For this review, take the finished solid that the model builds, in its own axes (mm). Face numbers are marked on the shaded views. A direction names the side the tool comes from. Coordinates: 2 decimals unless noted, no trailing zeros. Loops run counter-clockwise (first coordinate to the right, second up) from the corner with the lowest first, then second, coordinate; pieces in that order, holes last. Notation, with made-up numbers: M 15.25,-21.75 L 42.25,-21.75 A24 cw 42.25,10.25 Z; hole C 48.5,63 d9. An arc over 180 degrees is marked long. Write item = value, one per line.
from build123d import *

# Parameters (mm, degrees)
ESQUISSE1_W                       = 5.5
ESQUISSE1_H                       = 36
BOSS_EXTRU_1_DEPTH                = 10
ESQUISSE2_R                       = 1.7
ENL_V_MAT_EXTRU_1_DEPTH           = 4
ENL_V_MAT_EXTRU_2_DEPTH           = 3.5
ENL_V_MAT_EXTRU_2_DRAFT           = 5
ENL_V_MAT_EXTRU_2_PROFILE_2_DEPTH = 3.5
ENL_V_MAT_EXTRU_2_PROFILE_2_DRAFT = 5
ENL_V_MAT_EXTRU_2_PROFILE_3_DEPTH = 3.5
ENL_V_MAT_EXTRU_2_PROFILE_3_DRAFT = 5
ENL_V_MAT_EXTRU_2_PROFILE_4_DEPTH = 3.5
ENL_V_MAT_EXTRU_2_PROFILE_4_DRAFT = 5
ESQUISSE4_W                       = 9.5
ESQUISSE4_H                       = 5
BOSS_EXTRU_2_DEPTH                = 50
ESQUISSE5_W                       = 9.5
ESQUISSE5_H                       = 9.5
BOSS_EXTRU_3_DEPTH                = 32
CONG_1_R                          = 4.75


with BuildPart() as part:
    # Esquisse1 → Boss.-Extru.1 (new body)
    with BuildSketch(Plane.XY):
        Rectangle(ESQUISSE1_W, ESQUISSE1_H)
    extrude(amount=BOSS_EXTRU_1_DEPTH)

    # Esquisse2 → Enlèv. mat.-Extru.1 (cut)
    with BuildSketch(Plane(origin=(2.75, 0, 0), x_dir=(0, 0, -1), z_dir=(1, 0, 0))):
        with Locations((-4, 10)):
            Circle(ESQUISSE2_R)
        with Locations((-4, 2)):
            Circle(ESQUISSE2_R)
        with Locations((-4, -6)):
            Circle(ESQUISSE2_R)
        with Locations((-4, -14)):
            Circle(ESQUISSE2_R)
    extrude(amount=-ENL_V_MAT_EXTRU_1_DEPTH, mode=Mode.SUBTRACT)


with BuildPart() as enl_v_mat_extru_2_tool:
    # Esquisse3 → Enlèv. mat.-Extru.2 (with draft: the straight prism first)
    with BuildSketch(Plane(origin=(-2.75, 0, 0), x_dir=(0, 0, -1), z_dir=(1, 0, 0))):
        Polygon((-2.574135551, 4.901765653), (-5.800070547, 4.685717662), (-7.225934996, 1.783952009), (-5.425864449, -0.901765653), (-2.199929453, -0.685717662), (-0.774065004, 2.216047991), align=None)
    extrude(amount=ENL_V_MAT_EXTRU_2_DEPTH)
    # Enlèv. mat.-Extru.2: the draft: its side faces are tilted about the plane it starts from
    enl_v_mat_extru_2_sides = [enl_v_mat_extru_2_tool.faces().sort_by_distance(p)[0] for p in [
        (-1, 4.793741658, 4.187103049),
        (-1, 3.234834835, 6.513002771),
        (-1, 0.441093178, 6.325899723),
        (-1, -0.793741658, 3.812896951),
        (-1, 0.765165165, 1.486997229),
        (-1, 3.558906822, 1.674100277),
    ]]
    draft(enl_v_mat_extru_2_sides, Plane(origin=(-2.75, 0, 0), x_dir=(0, 0, -1), z_dir=(1, 0, 0)), ENL_V_MAT_EXTRU_2_DRAFT)


with BuildPart() as part_1:
    add(part.part)

    # Enlèv. mat.-Extru.2: cut by enl_v_mat_extru_2_tool
    add(enl_v_mat_extru_2_tool.part, mode=Mode.SUBTRACT)


with BuildPart() as enl_v_mat_extru_2_profile_2_tool:
    # Esquisse3 → Enlèv. mat.-Extru.2 profile 2 (with draft: the straight prism first)
    with BuildSketch(Plane(origin=(-2.75, 0, 0), x_dir=(0, 0, -1), z_dir=(1, 0, 0))):
        Polygon((-2.574135551, 12.901765653), (-5.800070547, 12.685717662), (-7.225934996, 9.783952009), (-5.425864449, 7.098234347), (-2.199929453, 7.314282338), (-0.774065004, 10.216047991), align=None)
    extrude(amount=ENL_V_MAT_EXTRU_2_PROFILE_2_DEPTH)
    # Enlèv. mat.-Extru.2 profile 2: the draft: its side faces are tilted about the plane it starts from
    enl_v_mat_extru_2_profile_2_sides = [enl_v_mat_extru_2_profile_2_tool.faces().sort_by_distance(p)[0] for p in [
        (-1, 12.793741658, 4.187103049),
        (-1, 11.234834835, 6.513002771),
        (-1, 8.441093178, 6.325899723),
        (-1, 7.206258342, 3.812896951),
        (-1, 8.765165165, 1.486997229),
        (-1, 11.558906822, 1.674100277),
    ]]
    draft(enl_v_mat_extru_2_profile_2_sides, Plane(origin=(-2.75, 0, 0), x_dir=(0, 0, -1), z_dir=(1, 0, 0)), ENL_V_MAT_EXTRU_2_PROFILE_2_DRAFT)


with BuildPart() as part_2:
    add(part_1.part)

    # Enlèv. mat.-Extru.2 profile 2: cut by enl_v_mat_extru_2_profile_2_tool
    add(enl_v_mat_extru_2_profile_2_tool.part, mode=Mode.SUBTRACT)


with BuildPart() as enl_v_mat_extru_2_profile_3_tool:
    # Esquisse3 → Enlèv. mat.-Extru.2 profile 3 (with draft: the straight prism first)
    with BuildSketch(Plane(origin=(-2.75, 0, 0), x_dir=(0, 0, -1), z_dir=(1, 0, 0))):
        Polygon((-2.574135551, -3.098234347), (-5.800070547, -3.314282338), (-7.225934996, -6.216047991), (-5.425864449, -8.901765653), (-2.199929453, -8.685717662), (-0.774065004, -5.783952009), align=None)
    extrude(amount=ENL_V_MAT_EXTRU_2_PROFILE_3_DEPTH)
    # Enlèv. mat.-Extru.2 profile 3: the draft: its side faces are tilted about the plane it starts from
    enl_v_mat_extru_2_profile_3_sides = [enl_v_mat_extru_2_profile_3_tool.faces().sort_by_distance(p)[0] for p in [
        (-1, -3.206258342, 4.187103049),
        (-1, -4.765165165, 6.513002771),
        (-1, -7.558906822, 6.325899723),
        (-1, -8.793741658, 3.812896951),
        (-1, -7.234834835, 1.486997229),
        (-1, -4.441093178, 1.674100277),
    ]]
    draft(enl_v_mat_extru_2_profile_3_sides, Plane(origin=(-2.75, 0, 0), x_dir=(0, 0, -1), z_dir=(1, 0, 0)), ENL_V_MAT_EXTRU_2_PROFILE_3_DRAFT)


with BuildPart() as part_3:
    add(part_2.part)

    # Enlèv. mat.-Extru.2 profile 3: cut by enl_v_mat_extru_2_profile_3_tool
    add(enl_v_mat_extru_2_profile_3_tool.part, mode=Mode.SUBTRACT)


with BuildPart() as enl_v_mat_extru_2_profile_4_tool:
    # Esquisse3 → Enlèv. mat.-Extru.2 profile 4 (with draft: the straight prism first)
    with BuildSketch(Plane(origin=(-2.75, 0, 0), x_dir=(0, 0, -1), z_dir=(1, 0, 0))):
        Polygon((-2.574135551, -11.098234347), (-5.800070547, -11.314282338), (-7.225934996, -14.216047991), (-5.425864449, -16.901765653), (-2.199929453, -16.685717662), (-0.774065004, -13.783952009), align=None)
    extrude(amount=ENL_V_MAT_EXTRU_2_PROFILE_4_DEPTH)
    # Enlèv. mat.-Extru.2 profile 4: the draft: its side faces are tilted about the plane it starts from
    enl_v_mat_extru_2_profile_4_sides = [enl_v_mat_extru_2_profile_4_tool.faces().sort_by_distance(p)[0] for p in [
        (-1, -11.206258342, 4.187103049),
        (-1, -12.765165165, 6.513002771),
        (-1, -15.558906822, 6.325899723),
        (-1, -16.793741658, 3.812896951),
        (-1, -15.234834835, 1.486997229),
        (-1, -12.441093178, 1.674100277),
    ]]
    draft(enl_v_mat_extru_2_profile_4_sides, Plane(origin=(-2.75, 0, 0), x_dir=(0, 0, -1), z_dir=(1, 0, 0)), ENL_V_MAT_EXTRU_2_PROFILE_4_DRAFT)


with BuildPart() as part_4:
    add(part_3.part)

    # Enlèv. mat.-Extru.2 profile 4: cut by enl_v_mat_extru_2_profile_4_tool
    add(enl_v_mat_extru_2_profile_4_tool.part, mode=Mode.SUBTRACT)

    # Esquisse4 → Boss.-Extru.2 (add)
    with BuildSketch(Plane.XY.offset(10)):
        with Locations((2, 2.5)):
            Rectangle(ESQUISSE4_W, ESQUISSE4_H)
    extrude(amount=BOSS_EXTRU_2_DEPTH)

    # Esquisse5 → Boss.-Extru.3 (add)
    with BuildSketch(Plane.XZ):
        with Locations((2, 55.25)):
            Rectangle(ESQUISSE5_W, ESQUISSE5_H)
    extrude(amount=BOSS_EXTRU_3_DEPTH)

    # Congé1
    cong_1_edges = [part_4.edges().sort_by_distance(p)[0] for p in [
        (-2.75, -32, 55.25),
        (2, -32, 50.5),
        (6.75, -32, 55.25),
        (2, -32, 60),
    ]]
    fillet(cong_1_edges, radius=CONG_1_R - 0.0001)  # a hair under: the kernel refuses the full size


solid = part_4.part
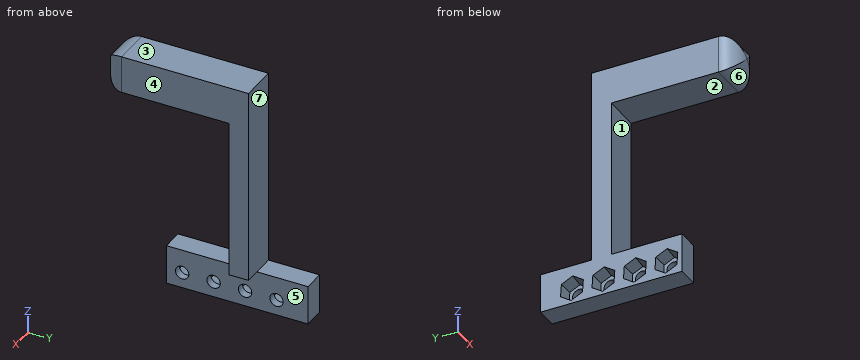
Q1. Draft analysis for pull direction Z (two halves, no side actions). For the marked faces 1, 2, 3 and 4, state which applies: +Z half, -Z half, draft (parallel to the pull), parting line (faces both ways), or undercut.
Solved:
face_1 = undercut
face_2 = undercut
face_3 = +Z half
face_4 = draft
Q2. Add section C-C (z = 52.5). Write out the cut boundary in (x, y), and give its area (3 significant figures).
Solved:
outline = M -2.75,-27.25 A4.75 ccw -0.75,-31.12 L 4.75,-31.12 A4.75 ccw 6.75,-27.25 L 6.75,5 L -2.75,5 Z
area = 339 mm²
Q3. For line 1 along Y through (x, z) = (1.5, 4); line 2 along Y through (x, z) = (1.5, 3); line 3 along Z through (x, y) = (-2, -10.5), list the stretches that pass through material, from the lowest coordinate up.
Solved:
line_1 = -18 to -15.7, -12.3 to -7.7, -4.3 to 0.3, 3.7 to 8.3, 11.7 to 18
line_2 = -18 to -15.37, -12.63 to -7.37, -4.63 to 0.63, 3.37 to 8.63, 11.37 to 18
line_3 = 0 to 10, 50.5 to 60
Q4. For pin 1 Ø1 at (x, z) = (1.5, 11.5) entering from -Y; pin 2 Ø3 at (y, z) = (-6, 4) entering from -X; pin 3 Ø1 at (x, y) = (-0.5, 6.5) entering from +Z; pin 4 Ø1.6 at (y, z) = (1, 3) entering from -X, all flat-tipped, find the tip position at first contact; note any pin that passes through.
Solved:
pin_1 = 0
pin_2 = through
pin_3 = 10
pin_4 = 0.75
Q5. Machinability: for the marked faces 5, 6 and 7, which of the approach directions +Z, -Z, +X, -X, +Y, -Y give a long, thin tool a straight path to every point of the face, cutting with its end or side? Answer none if there is none.
Solved:
face_5 = -Z, +X, +Y, -Y
face_6 = -Z, +X, -X, -Y
face_7 = +Z, +X, -X, +Y
Q6. Add section D-D (x = -0.25). State how many separate pieces and enclosed holes the cut face has, and give its area (3 significant figures).
Solved:
separate_pieces = 1
enclosed_holes = 4
area = 810 mm²
Q7. Add section B-B (x = 3.5). Write out the cut boundary in (y, z).
Solved:
outline = M -31.76,53.75 A4.75 ccw -27.25,50.5 L 0,50.5 L 0,10 L 5,10 L 5,60 L -27.25,60 A4.75 ccw -31.76,56.75 Z
Q8. Add section A-A (y = -21.5). Write out the cut boundary in (x, z).
Solved:
outline = M -2.75,50.5 L 6.75,50.5 L 6.75,60 L -2.75,60 Z
